Study the drawing (mm; zero at the part's minimum x, y, z) and answer. Coordinates: 2 decimals unless noted, no trailing zeros. Order: outer loops, then holes, each group sorted by start corner. A loop starts at its lowest first (then second) coordinate and runs counter-clockwise, first axis right, second up. Notation, with made-up numbers: (73, -30.75) -> (89, -30.75) arc R27 ccw to (89, -5.75) -> close; hole circle Ø2 at (-34.75, -25.5). An arc over 180 degrees is marked (long way). Answer as CSV lines item,"result". Start each with the question number.
Item 1: Section C-C (y = 1.1) is taken. Count the separate pieces of the cut face and the enclosed holes in it, then the cut area to 3 significant figures.
Item 2: Section D-D (x = 32) is taken. Write down the section's boundary in (y, z), then the cut area to 3 significant figures.
Item 3: Section A-A (z = 43.25) is taken. Write down the section's boundary in (x, y), then the cut area to 3 significant figures.
Item 4: Straight lines are drawn through the part: L1, parallel to X at y = 1.65, z = 3.75; L2, parallel to X at y = 1.2, z = 44; L3, parallel to Z at x = 53.5, y = 1.25. For each, find the intervals that lie inside material, in ascending order.
Item 5: Section B-B (x = 51.9) is taken. Write down the section's boundary in (y, z).
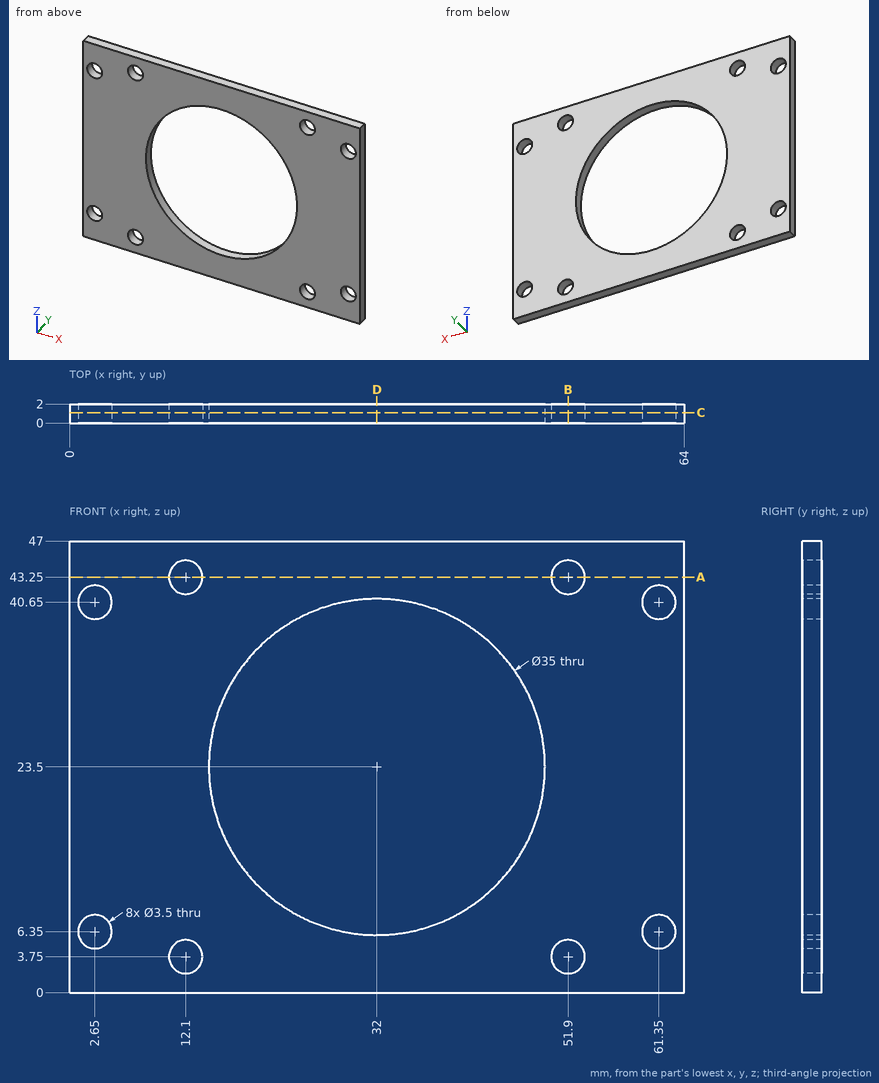
Checked values:
1,separate pieces,"1"
1,enclosed holes,"9"
1,area,"1,970 mm^2"
2,outline,"(0, 0) -> (2, 0) -> (2, 6) -> (0, 6) -> close; (0, 41) -> (2, 41) -> (2, 47) -> (0, 47) -> close"
2,area,"24.0 mm^2"
3,outline,"(0, 0) -> (10.35, 0) -> (10.35, 2) -> (0, 2) -> close; (13.85, 0) -> (50.15, 0) -> (50.15, 2) -> (13.85, 2) -> close; (53.65, 0) -> (64, 0) -> (64, 2) -> (53.65, 2) -> close"
3,area,"114 mm^2"
4,L1,"x = 0 to 10.35, 13.85 to 50.15, 53.65 to 64"
4,L2,"x = 0 to 10.52, 13.68 to 50.32, 53.48 to 64"
4,L3,"z = 0 to 3.04, 4.46 to 42.54, 43.96 to 47"
5,outline,"(0, 0) -> (2, 0) -> (2, 2) -> (0, 2) -> close; (0, 5.5) -> (2, 5.5) -> (2, 41.5) -> (0, 41.5) -> close; (0, 45) -> (2, 45) -> (2, 47) -> (0, 47) -> close"
